Check sheet for the modelled part. Datum: model origin and axes. Units: mm. A direction names the side the tool comes from. Coordinates: 2 decimals unless noted, no trailing zeros. Write each loop counter-clockwise with the first axis right and the second up, starting at its lowest first coordinate (ties: lowest second). Pieces come first, ordered by that corner, then holes. Notation, with made-up numbers: (72.5, 7) - (104.5, 7) arc R4 cw to (104.5, 13) - close; hole circle Ø11 at (-15, 49.5). An arc over 180 degrees is marked (long way). Use one line per item in the form item = value. Start each with the question number.
1. Scan lines: line 1 along Y through (x, z) = (-50.75, 10); line 2 along X through (y, z) = (113, 13); line 3 along X through (y, z) = (75.5, 18.5). Record each from-to range of solid material in increasing order.
2. Draft check along Z on faces 4 (the face through (16, 15.099, 10)), 5 (the face through (-52.7, 55, 10)), 6 (the face through (0, 112, 20)), 7 (the face through (-52.73, 35.663, 7.693)). Enter one of: +Z half, -Z half, draft (parallel to the pull), parting line (faces both ways), or undercut.
3. Cross-section at B-B on y = 48. Record the boundary of the cut face in (x, z).
4. Go/stop test with flat-tipped pins: pin 1 Ø6 at (y, z) = (72.6, 10) entering from -X; pin 2 Ø8 at (y, z) = (28.5, 13.5) entering from -X; pin 3 Ø5 at (y, z) = (23.5, 9) entering from -X. Record where each tip stops, or that it passes through.
5. Tool access check on faces 1 (the face through (41, 118.654, 10)), 2 (the face through (0, 112, 0)), 3 (the face through (-52.73, 29.315, 7.312)). Record the directions out of +Z, -Z, +X, -X, +Y, -Y that give a thin tool (end or side, any length) a straight path to the whole face; none if there is none.
6. Cross-section at C-C on y = 88. Record the boundary of the cut face in (x, z).
7. Cross-section at A-A on x = 19. Record the boundary of the cut face in (y, z).
```python
from build123d import *

# Parameters (mm, degrees)
SKETCH_4_W          = 150
SKETCH_4_H          = 115
EXTRUDE_1_DEPTH     = 20
CUT_EXTRUDE_1_DEPTH = 20
SKETCH_6_R          = 5
CUT_EXTRUDE_7_DEPTH = 10
SKETCH_9_R          = 5
CUT_EXTRUDE_8_DEPTH = 5
SKETCH_11_R         = 5
CUT_EXTRUDE_9_DEPTH = 5


with BuildPart() as part:
    # 草圖4 → 填料-伸長1 (new body)
    with BuildSketch(Plane.XY):
        with Locations((17.378483322, 72.59909222)):
            Rectangle(SKETCH_4_W, SKETCH_4_H)
    extrude(amount=EXTRUDE_1_DEPTH)

    # 草圖2 → 除料-伸長1 (cut)
    with BuildSketch(Plane.XY):
        with BuildLine():
            Line((-47.207745562, 65.711609892), (-47.207745562, 79.486574548))
            ThreePointArc((-47.207745562, 79.486574548), (-45.199499918, 87.30172842), (-39.672345291, 93.180524415))
            ThreePointArc((-39.672345291, 93.180524415), (-34.318944815, 96.349970124), (-28.784309893, 99.191114091))
            ThreePointArc((-28.784309893, 99.191114091), (-15.358686248, 104.775217116), (-1.443024263, 108.992316634))
            ThreePointArc((-1.443024263, 108.992316634), (5.275172672, 110.237187628), (12.094993869, 110.654216049))
            Line((12.094993869, 110.654216049), (33.772014803, 110.654216049))
            Line((33.772014803, 110.654216049), (36.848505718, 110.654216049))
            Line((36.848505718, 110.654216049), (36.848505718, 118.654216049))
            Line((36.848505718, 118.654216049), (44.287834674, 118.654216049))
            Line((44.287834674, 118.654216049), (44.287834674, 112.450982223))
            Line((44.287834674, 112.450982223), (45.736024045, 112.450982223))
            Line((45.736024045, 112.450982223), (45.736024045, 122.450982223))
            Line((45.736024045, 122.450982223), (50.704341659, 122.450982223))
            Line((50.704341659, 122.450982223), (50.704341659, 112.450982223))
            Line((50.704341659, 112.450982223), (51.627972578, 112.450982223))
            Line((51.627972578, 112.450982223), (51.627972578, 119.746473649))
            Line((51.627972578, 119.746473649), (57.89832581, 119.746473649))
            Line((57.89832581, 119.746473649), (57.89832581, 111.746473649))
            ThreePointArc((57.89832581, 111.746473649), (67.349215797, 109.578876862), (74.910898446, 103.509383234))
            ThreePointArc((74.910898446, 103.509383234), (75.840394113, 102.31020351), (76.746696007, 101.093399876))
            ThreePointArc((76.746696007, 101.093399876), (83.438828083, 89.130434251), (87.081135301, 75.915640404))
            Line((87.081135301, 75.915640404), (87.182187493, 75.239707939))
            ThreePointArc((87.182187493, 75.239707939), (87.378483322, 72.59909222), (87.182187493, 69.958476501))
            Line((87.182187493, 69.958476501), (87.081135301, 69.282544036))
            ThreePointArc((87.081135301, 69.282544036), (83.438828083, 56.06775019), (76.746696007, 44.104784564))
            ThreePointArc((76.746696007, 44.104784564), (75.840394113, 42.887980931), (74.910898446, 41.688801206))
            ThreePointArc((74.910898446, 41.688801206), (67.349215797, 35.619307578), (57.89832581, 33.451710791))
            Line((57.89832581, 33.451710791), (57.89832581, 25.451710791))
            Line((57.89832581, 25.451710791), (51.627972578, 25.451710791))
            Line((51.627972578, 25.451710791), (51.627972578, 32.747202217))
            Line((51.627972578, 32.747202217), (50.704341659, 32.747202217))
            Line((50.704341659, 32.747202217), (50.704341659, 22.747202217))
            Line((50.704341659, 22.747202217), (45.736024045, 22.747202217))
            Line((45.736024045, 22.747202217), (45.736024045, 32.747202217))
            Line((45.736024045, 32.747202217), (44.287834674, 32.747202217))
            Line((44.287834674, 32.747202217), (44.287834674, 26.543968391))
            Line((44.287834674, 26.543968391), (36.848505718, 26.543968391))
            Line((36.848505718, 26.543968391), (36.848505718, 34.543968391))
            Line((36.848505718, 34.543968391), (33.772014803, 34.543968391))
            Line((33.772014803, 34.543968391), (12.094993869, 34.543968391))
            ThreePointArc((12.094993869, 34.543968391), (5.275172672, 34.960996812), (-1.443024263, 36.205867806))
            ThreePointArc((-1.443024263, 36.205867806), (-15.358686248, 40.422967325), (-28.784309893, 46.007070349))
            ThreePointArc((-28.784309893, 46.007070349), (-34.318944815, 48.848214316), (-39.672345291, 52.017660026))
            ThreePointArc((-39.672345291, 52.017660026), (-45.199499918, 57.89645602), (-47.207745562, 65.711609892))
        make_face()
    extrude(amount=CUT_EXTRUDE_1_DEPTH, mode=Mode.SUBTRACT)

    # 草圖6 → 除料-伸長7 (cut)
    with BuildSketch(Plane(origin=(-57.7, 0, 0), x_dir=(0, 0, -1), z_dir=(1, 0, 0))):
        with Locations((-10, 120.09909222)):
            Circle(SKETCH_6_R)
        with Locations((-10, 105.09909222)):
            Circle(SKETCH_6_R)
        with Locations((-10, 40.09909222)):
            Circle(SKETCH_6_R)
        with Locations((-10, 25.09909222)):
            Circle(SKETCH_6_R)
    extrude(amount=CUT_EXTRUDE_7_DEPTH, mode=Mode.SUBTRACT)

    # 草圖9 → 除料-伸長8 (cut)
    with BuildSketch(Plane(origin=(-57.7, 0, 0), x_dir=(0, 0, -1), z_dir=(1, 0, 0))):
        with Locations((-10, 90.09909222)):
            Circle(SKETCH_9_R)
        with Locations((-10, 55.09909222)):
            Circle(SKETCH_9_R)
    extrude(amount=CUT_EXTRUDE_8_DEPTH, mode=Mode.SUBTRACT)

    # 草圖11 → 除料-伸長9 (cut)
    with BuildSketch(Plane(origin=(-57.7, 0, 0), x_dir=(0, 0, -1), z_dir=(1, 0, 0))):
        with Locations((-10, 72.59909222)):
            Circle(SKETCH_11_R)
    extrude(amount=CUT_EXTRUDE_9_DEPTH, mode=Mode.SUBTRACT)


solid = part.part
```
Final values:
q1.line_1 = 15.1 to 20.1, 30.1 to 35.1, 45.1 to 100.1, 110.1 to 115.1, 125.1 to 130.1
q1.line_2 = -57.62 to 36.85, 44.29 to 45.74, 50.7 to 51.63, 57.9 to 92.38
q1.line_3 = -57.62 to -47.21, 87.14 to 92.38
q2.face_4 = draft
q2.face_5 = undercut
q2.face_6 = +Z half
q2.face_7 = undercut
q3.outline = (-57.62, 0) - (-32.75, 0) - (-32.75, 20) - (-57.62, 20) - close; (79.35, 0) - (92.38, 0) - (92.38, 20) - (79.35, 20) - close
q4.pin_1 = -52.7
q4.pin_2 = -57.62
q4.pin_3 = -47.7
q5.face_1 = +Z, -Z
q5.face_2 = -Z, +X, -X, +Y, -Y
q5.face_3 = -X
q6.outline = (-57.62, 0) - (-44.79, 0) - (-44.79, 20) - (-57.62, 20) - (-57.62, 14.54) - (-52.7, 14.54) - (-52.7, 5.46) - (-57.62, 5.46) - close; (83.89, 0) - (92.38, 0) - (92.38, 20) - (83.89, 20) - close
q7.outline = (15.1, 0) - (34.54, 0) - (34.54, 20) - (15.1, 20) - close; (110.65, 0) - (130.1, 0) - (130.1, 20) - (110.65, 20) - close
